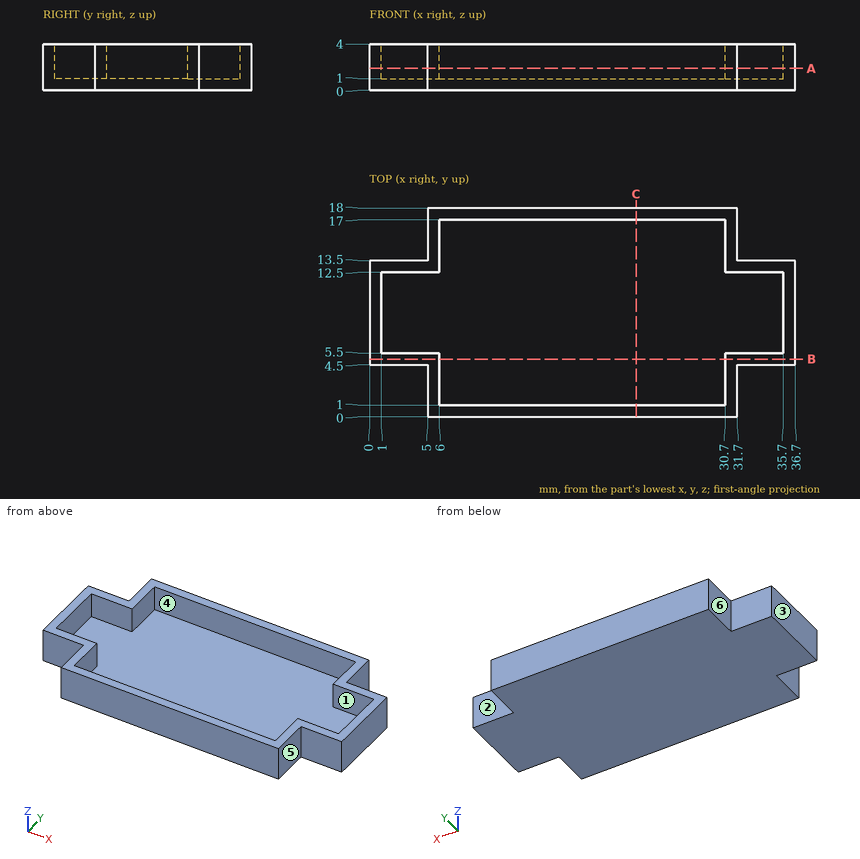
Source: three-view drawing plus pictorial views. Frame: mm from the lowest corner of the part. A direction names the side the tool comes from. Coordinates: 2 decimals unless noted, no trailing zeros. Loops run counter-clockwise (first coordinate to the right, second up) from the corner with the lowest first, then second, coordinate; pieces in that order, holes last. Notation, with made-up numbers: (-33, 18.25) - (9, 18.25) arc R6 ccw to (9, 27.25) - close; hole circle Ø4 at (54, 42.5). An arc over 180 degrees is marked (long way). One line per question, with ' | ' between items.
1) Section C-C, the plane x = 23. Return loops of the section in (y, z), then the cut area to 3 significant figures.
Report:
outline: (0, 0) - (18, 0) - (18, 4) - (17, 4) - (17, 1) - (1, 1) - (1, 4) - (0, 4) - close | area: 24.0 mm²
2) Pull-direction query (Y, two-part tool) for the marked faces 1, 2 and 3; classes: released by +Y, released by -Y, zero draft, split by the parting line, or undercut.
Report:
face 1: undercut | face 2: released by +Y | face 3: zero draft
3) Line query: line 1 along Y through (x, z) = (23.5, 2.55); line 2 along X through (y, z) = (7.5, 2.65); line 3 along X through (y, z) = (1.25, 1.5). Output: solid intervals per line, ascending.
Report:
line 1: y = 0 to 1, 17 to 18 | line 2: x = 0 to 1, 35.7 to 36.7 | line 3: x = 5 to 6, 30.7 to 31.7
4) Section B-B, the plane y = 5. Return loops of the section in (x, z), then the cut area to 3 significant figures.
Report:
outline: (0, 0) - (36.7, 0) - (36.7, 4) - (30.7, 4) - (30.7, 1) - (6, 1) - (6, 4) - (0, 4) - close | area: 72.7 mm²
5) First-contact query: P1, Ø0.9, axis at x = 33.5, z = 3, coming from the +Y side; P2, Ø1.5, axis at y = 15.5, z = 2, coming from the -X side; P3, Ø1.5, axis at x = 34, z = 2.5, coming from the -Y side. Flat tips, straight axial feed; report the tip coordinate or a pass-through.
Report:
P1: stops at y = 13.5 | P2: stops at x = 5 | P3: stops at y = 4.5
6) Section A-A, the plane z = 1.9. Return loops of the section in (x, y).
Report:
outline: (0, 4.5) - (5, 4.5) - (5, 0) - (31.7, 0) - (31.7, 4.5) - (36.7, 4.5) - (36.7, 13.5) - (31.7, 13.5) - (31.7, 18) - (5, 18) - (5, 13.5) - (0, 13.5) - close; hole (1, 5.5) - (6, 5.5) - (6, 1) - (30.7, 1) - (30.7, 5.5) - (35.7, 5.5) - (35.7, 12.5) - (30.7, 12.5) - (30.7, 17) - (6, 17) - (6, 12.5) - (1, 12.5) - close
7) Set-up query: the marked faces 4, 5 and 6. Return all of +Z, -Z, +X, -X, +Y, -Y with unobstructed straight access to the full face (end or side cutting, diameter ignored); none if empty.
Report:
face 4: +Z | face 5: +Z, -Z, +X, -Y | face 6: +Z, -Z, -X, +Y
